Study the drawing (mm; zero at the part's minimum x, y, z) and answer. A direction names the side the tool comes from. Coordinates: 2 decimals unless noted, no trailing zeros. Loops run counter-clockwise (first coordinate to the right, second up) from the corner with the lowest first, then second, coordinate; pieces in that order, holes last. Notation, with made-up numbers: M 81,45 L 93,45 A34 ccw 93,78 Z; hole C -19.75,-3.75 d3. An arc over 180 degrees is marked long. Use one line per item in the form item = value. Start each with the question number.
1. The part is cut by section A-A (z = 13.5). Give the vertices of the cut face in (x, y).
2. A tool of negligible diameter and unlimited length cuts with its end or side. For the marked faces 1, 2 and 3, from which of +Z, -Z, +X, -X, +Y, -Y can it reach the whole face along a straight path? Write none if from no direction.
3. The part is cut by section D-D (y = 12). Give the vertices of the cut face in (x, z).
4. Flat-ended cylindrical pins translate along their axes: pin 1 (3 mm diameter, centred on x = 25, z = 29.5, fed in from +Y); pin 2 (2.5 mm diameter, centred on x = 19.5, y = 2, fed in from +Z); pin 3 (1 mm diameter, centred on x = 30, y = 19, fed in from +Z). Find the tip coordinate at first contact, or state that the pin passes through.
5. The part is cut by section B-B (x = 20). Give the vertices of the cut face in (y, z), plus the area to 3 significant figures.
6. The part is cut by section C-C (z = 36). Give the vertices of the cut face in (x, y), plus the area to 3 significant figures.
7. For a pull along Z with two mould halves and no side action, classify the marked faces 4, 5 and 6 as released by +Z, released by -Z, zero draft, split by the parting line, or undercut.
8. Find the intervals of material crossed by probe 1 along Y at (x, z) = (9, 17.5); probe 2 along Y at (x, z) = (15, 33); probe 3 along Z at (x, y) = (11, 44), in increasing order. Write a range as [from, to].
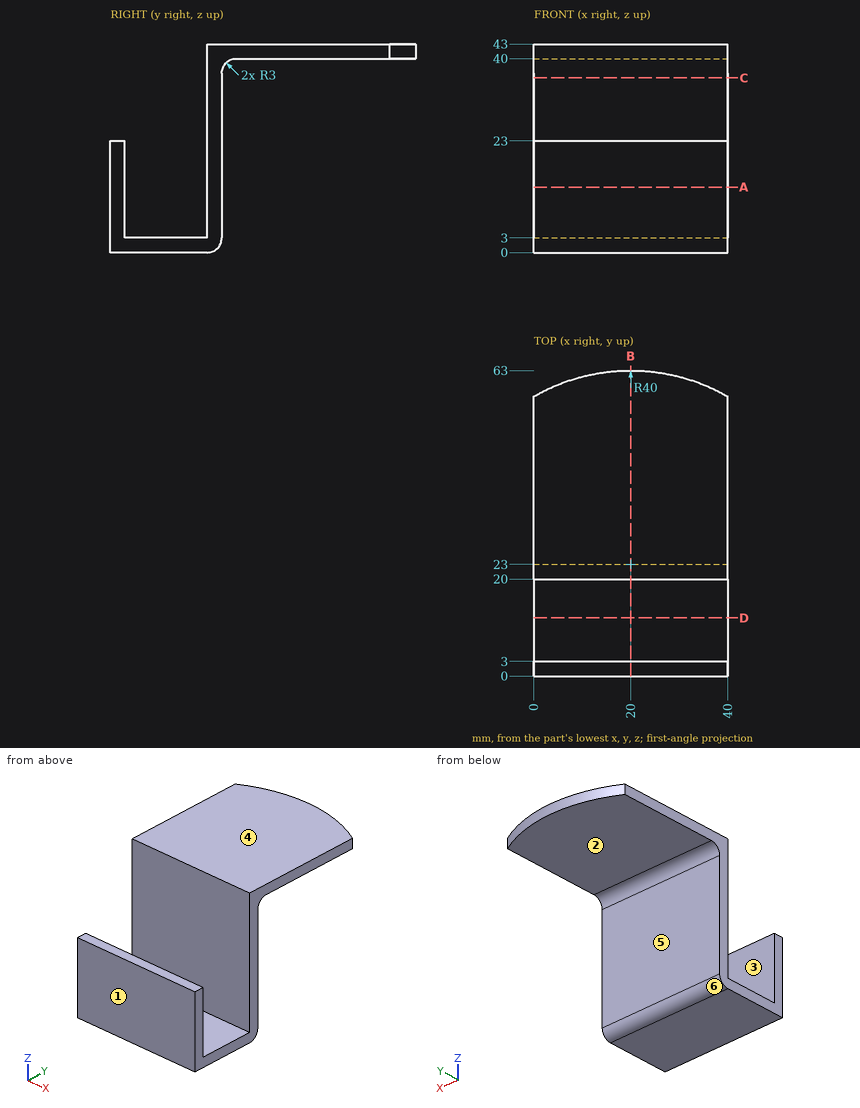
Computed values:
q1.outline = M 0,0 L 40,0 L 40,3 L 0,3 Z; M 0,20 L 40,20 L 40,23 L 0,23 Z
q2.face_1 = +Z, -Z, +X, -X, -Y
q2.face_2 = -Z, +X, -X, +Y
q2.face_3 = +Z, +X, -X
q3.outline = M 0,0 L 40,0 L 40,3 L 0,3 Z
q4.pin_1 = 23
q4.pin_2 = 23
q4.pin_3 = 3
q5.outline = M 0,0 L 20,0 A3 ccw 23,3 L 23,37 A3 cw 26,40 L 63,40 L 63,43 L 20,43 L 20,3 L 3,3 L 3,23 L 0,23 Z
q5.area = 369 mm²
q6.outline = M 0,20 L 40,20 L 40,23 L 0,23 Z
q6.area = 120 mm²
q7.face_4 = released by +Z
q7.face_5 = zero draft
q7.face_6 = released by -Z
q8.probe_1 = [0, 3], [20, 23]
q8.probe_2 = [20, 23]
q8.probe_3 = [40, 43]
